The figure shows three views and two pictorial views of one solid part (mm, origin at its lowest corner). Answer the questions. Coordinates: 2 decimals unless noted, no trailing zeros. Answer in a Markdown table with one row per item. Add a question column.
Item 1: The mould has two halves that part along Y. Classify the marked faces 1, 2 and 3: released by +Y, released by -Y, zero draft, split by the parting line, or undercut.
Item 2: Consider line 1 (Y direction, x = 4, z = 2.1) (1 decimal); line 2 (X direction, y = 8.75, z = 2.4) (1 decimal); line 3 (Y direction, x = 5.75, z = 0.6) (1 decimal). Determine where each line is inside the solid, lowest interval first. Write a range as from..to.
Item 3: A flat-ended cylindrical pin translates along its axis: pin 1 Ø1 at (x, z) = (8, 3.5) entering from +Y. Find the tip coordinate at first contact, or state that the pin passes through.
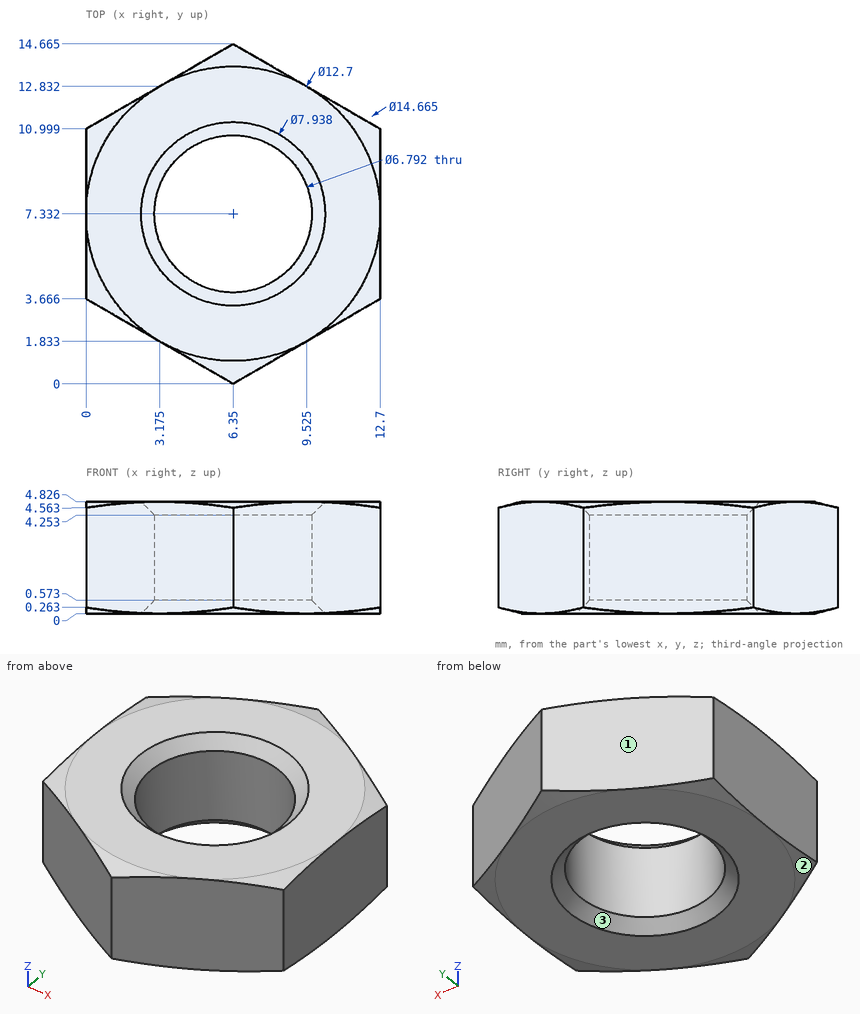
Reply:
| question | item | result |
|---|---|---|
| 1 | face 1 | released by +Y |
| 1 | face 2 | released by -Y |
| 1 | face 3 | undercut |
| 2 | line 1 | y = 1.4..4.9, 9.8..13.3 |
| 2 | line 2 | x = 0..3.3, 9.4..12.7 |
| 2 | line 3 | y = 0.3..4, 10.7..14.3 |
| 3 | pin 1 | stops at y = 14 |
